Source: CAD feature listing. Evaluate the final solid. Frame: model axes, mm. A direction names the side the tool comes from. Give positions to 0.01 mm unless a question says otherwise; leave off trailing zeros. Order: outer loops, then holes, each group sorted by start corner. A loop starts at its lowest first (then second) coordinate and runs counter-clockwise, first axis right, second up.
1) Section B-B, the plane z = -255.5. Return loops of the section in (x, y), plus the area to 3 significant figures.
2) Material intervals for line 1 (Y direction, x = 300, z = -141.5); line 2 (X direction, y = -248, z = -160); line 3 (Z direction, x = 243, y = -199.5), sorted ascending.
3) First-contact query: P1, Ø5, axis at y = 319, z = -244, coming from the -X side; P2, Ø1, axis at y = 205.5, z = 145.5, coming from the +X side. Flat tips, straight axial feed; report the tip coordinate or a pass-through.
4) Access query for faces 1 (the face through (-238, 0, 5)), 2 (the face through (-549, -241, -150)), 3 (the face through (-500, -115, -3)), 4 (the face through (-8, -300, -249)). Directions: +Z, -Z, +X, -X, +Y, -Y. A direction counts if a zero-diameter tool reaches every point of the face in a straight line with its end or side. Return the directions, or none.
5) Draft query along Z for faces 5 (the face through (452.6, 148.1, 4.9)), 6 (the face through (125, -20, 350)), 7 (the face through (186, -241, 150)), 8 (the face through (-549, -241, 150)). Return one class per face: released by +Z, released by -Z, zero draft, split by the parting line, or undercut.
6) Section C-C, the plane y = -131. Return loops of the section in (x, z).
7) Section D-D, the plane y = 14. Return loops of the section in (x, z), plus the area to 3 significant figures.
8) Section A-A, the plane x = 300. Return loops of the section in (y, z), plus the area to 3 significant figures.
```python
from build123d import *

# Parameters (mm, degrees)
F0_W      = 1200
F0_H      = 700
F1_DEPTH  = 300
F3_DEPTH  = 700
F5_W      = 240
F5_H      = 300
F6_DEPTH  = 1200.001
F7_W      = 260
F7_H      = 460
F8_DEPTH  = 300.001
F9_R      = 50
F10_R     = 160
F11_DEPTH = 700.001


with BuildPart() as f1:
    # F0 (on Front) → F1 (new body)
    with BuildSketch(Plane.XZ):
        Rectangle(F0_W, F0_H)
    extrude(amount=F1_DEPTH)

    # F2 (on face) → F3 (join)
    with BuildSketch(Plane.XY.offset(350)):
        with BuildLine():
            Line((0, 108.350513), (0, 0))
            Line((0, 0), (600, 0))
            Line((600, 0), (600, 108.350513))
            ThreePointArc((600, 108.350513), (300, 408.350513), (0, 108.350513))
        make_face()
    extrude(amount=-F3_DEPTH)

    # F5 (on face) → F6 (cut, through all)
    with BuildSketch(Plane.YZ.offset(600)):
        with Locations((-300, 0)):
            Rectangle(F5_W, F5_H)
    extrude(amount=-F6_DEPTH, mode=Mode.SUBTRACT)

    # F7 (on face) → F8 (cut, through all)
    with BuildSketch(Plane(origin=(0, 0, 0), x_dir=(-1, 0, 0), z_dir=(0, 1, 0))):
        with Locations((370, 0)):
            Rectangle(F7_W, F7_H)
    extrude(amount=-F8_DEPTH, mode=Mode.SUBTRACT)

    # F9
    f9_edges = [f1.edges().sort_by_distance(p)[0] for p in [
        (-240, -150, -230),
        (-240, -150, 230),
        (-500, -150, 230),
        (-500, -150, -230),
    ]]
    fillet(f9_edges, radius=F9_R)

    # F10 (on face) → F11 (cut, through all)
    with BuildSketch(Plane.XY.offset(350)):
        with Locations((300, 100)):
            Circle(F10_R)
    extrude(amount=-F11_DEPTH, mode=Mode.SUBTRACT)


solid = f1.part
```
From the geometry:
1. outline: (-600, -300) - (600, -300) - (600, 108.35) arc R300 ccw to (0, 108.35) - (0, 0) - (-600, 0) - close; hole circle Ø320 at (300, 100)
1. area: 486,000 mm2
2. line 1: y = -180 to -60, 260 to 408.35
2. line 2: x = -600 to -500, -240 to 600
2. line 3: z = -350 to -150, 150 to 350
3. P1: stops at x = 83.96
3. P2: stops at x = 584.01
4. face 1: +Z, -Z, -X, +Y
4. face 2: +X, -X, -Y
4. face 3: +Y, -Y
4. face 4: +Z, -Z, +X, -X, -Y
5. face 5: zero draft
5. face 6: released by +Z
5. face 7: undercut
5. face 8: undercut
6. outline: (-600, -350) - (600, -350) - (600, 350) - (-600, 350) - close; hole (-500, -180) arc R50 ccw to (-450, -230) - (-290, -230) arc R50 ccw to (-240, -180) - (-240, 180) arc R50 ccw to (-290, 230) - (-450, 230) arc R50 ccw to (-500, 180) - close
7. outline: (0, -350) - (165.08, -350) - (165.08, 350) - (0, 350) - close; (434.92, -350) - (600, -350) - (600, 350) - (434.92, 350) - close
7. area: 231,000 mm2
8. outline: (-300, -350) - (-60, -350) - (-60, 350) - (-300, 350) - (-300, 150) - (-180, 150) - (-180, -150) - (-300, -150) - close; (260, -350) - (408.35, -350) - (408.35, 350) - (260, 350) - close
8. area: 236,000 mm2
